```python
from build123d import *

# Parameters (mm, degrees)
F0_R      = 14
F1_DEPTH  = 15
F2_R      = 3
F3_DEPTH  = 50
F6_DEPTH  = 19.3
F7_DEPTH  = 19.3
F9_DEPTH  = 25
F10_DEPTH = 25


with BuildPart() as f1:
    # F0 (on Front) → F1 (new body)
    with BuildSketch(Plane.XZ):
        with BuildLine():
            Line((0, 44), (-94, 44))
            ThreePointArc((-94, 44), (-116, 22), (-94, 0))
            Line((-94, 0), (0, 0))
            ThreePointArc((0, 0), (22, 22), (0, 44))
        make_face()
        with BuildLine():
            Line((-105.5, 13), (-103.5, 13))
            ThreePointArc((-103.5, 13), (-101, 10.5), (-103.5, 8))
            Line((-103.5, 8), (-105.5, 8))
            ThreePointArc((-105.5, 8), (-108, 10.5), (-105.5, 13))
        make_face(mode=Mode.SUBTRACT)
        with BuildLine():
            Line((-84.5, 14), (-82.5, 14))
            ThreePointArc((-82.5, 14), (-80, 11.5), (-82.5, 9))
            Line((-82.5, 9), (-84.5, 9))
            ThreePointArc((-84.5, 9), (-87, 11.5), (-84.5, 14))
        make_face(mode=Mode.SUBTRACT)
        with BuildLine():
            Line((-96, 27), (-92, 27))
            ThreePointArc((-92, 27), (-87, 22), (-92, 17))
            Line((-92, 17), (-96, 17))
            ThreePointArc((-96, 17), (-100.999999, 22), (-96, 27))
        make_face(mode=Mode.SUBTRACT)
        with BuildLine():
            Line((-105.5, 35), (-103.5, 35))
            ThreePointArc((-103.5, 35), (-101, 32.5), (-103.5, 30))
            Line((-103.5, 30), (-105.5, 30))
            ThreePointArc((-105.5, 30), (-108, 32.5), (-105.5, 35))
        make_face(mode=Mode.SUBTRACT)
        with BuildLine():
            Line((-84.5, 35), (-82.5, 35))
            ThreePointArc((-82.5, 35), (-80, 32.5), (-82.5, 30))
            Line((-82.5, 30), (-84.5, 30))
            ThreePointArc((-84.5, 30), (-87, 32.5), (-84.5, 35))
        make_face(mode=Mode.SUBTRACT)
        with Locations((0, 22)):
            Circle(F0_R, mode=Mode.SUBTRACT)
    extrude(amount=-F1_DEPTH)

    # F2 (on Top) → F3 (cut)
    with BuildSketch(Plane.XY):
        with Locations((0, 7.5)):
            Circle(F2_R)
    extrude(amount=F3_DEPTH, mode=Mode.SUBTRACT)

    # F5 (on offset) → F6 (cut)
    with BuildSketch(Plane.XY.offset(22)):
        Polygon((4.767146, 4.243061), (5.204165, 10), (0.437019, 13.256939), (-4.767146, 10.756939), (-5.204165, 5), (-0.437019, 1.743061), align=None)
    extrude(amount=F6_DEPTH, mode=Mode.SUBTRACT)

    # F5 (on offset) → F7 (cut)
    with BuildSketch(Plane.XY.offset(22)):
        Polygon((4.767146, 4.243061), (5.204165, 10), (0.437019, 13.256939), (-4.767146, 10.756939), (-5.204165, 5), (-0.437019, 1.743061), align=None)
    extrude(amount=-F7_DEPTH, mode=Mode.SUBTRACT)

    # F8 (on offset) → F9 (cut)
    with BuildSketch(Plane.XY.offset(22)):
        Polygon((-116, 15), (-116, 7.5), (-66, 7.5), (-31, 15), align=None)
    extrude(amount=-F9_DEPTH, mode=Mode.SUBTRACT)

    # F8 (on offset) → F10 (cut)
    with BuildSketch(Plane.XY.offset(22)):
        Polygon((-116, 15), (-116, 7.5), (-66, 7.5), (-31, 15), align=None)
    extrude(amount=F10_DEPTH, mode=Mode.SUBTRACT)


solid = f1.part
```
For this review, take the finished solid that the model builds, in its own axes (mm). A direction names the side the tool comes from. Coordinates: 2 decimals unless noted, no trailing zeros. Loops run counter-clockwise (first coordinate to the right, second up) from the corner with the lowest first, then second, coordinate; pieces in that order, holes last.
1. Insertion check: P1, Ø2, axis at x = -99.5, z = 23, coming from the -Y side; P2, Ø5, axis at y = 2, z = 29, coming from the -X side; P3, Ø0.6, axis at x = -105, y = 2.5, coming from the -Z side; P4, Ø5, axis at x = -101, z = 23.5, coming from the +Y side. Each pin has a flat end and moves straight along its axis. Give the tip position at first contact, or say it passes through.
2. Add section D-D, the plane z = 39. Give the boundary of the cut face in (x, y), then the cut area to 3 significant figures.
3. Add section A-A, the plane z = 22. Give the boundary of the cut face in (x, y), then the cut area to 3 significant figures.
4. For line 1 (Y direction, x = 0, z = 1); line 2 (X direction, y = 5.5, z = 26); line 3 (Y direction, x = -4.5, z = 38), list the stretches that pass through material, from the lowest coordinate up.
5. Mouldability with a two-part tool opening along Y and no side actions: class faces 1 (the flat face through (4.983, 7.081, 38.104)), 2 (the flat face through (-37, 6, 0)), 3 (the flat face through (-48, 0, 22)) as +Y half, -Y half, draft (parallel to the pull), parting line (faces both ways), or undercut.
6. For faces 4 (the flat face through (2, 5, 41.3)), 5 (the cylindrical face through (-101, 4, 22)), 6 (the cylindrical face through (-3, 7.6, 42.6)), list the 3-axis set-ups (+Z, -Z, +X, -X, +Y, -Y) from which the entire face can be reached by the end or side of a thin tool; tool diameter is ignored.
7. Add section B-B, the plane z = 11.5. Give the boundary of the cut face in (x, y), then the cut area to 3 significant figures.
8. Add section C-C, the plane x = -59. Give the boundary of the cut face in (y, z), then the cut area to 3 significant figures.
Result:
1. P1: passes through
1. P2: stops at x = -115.53
1. P3: stops at z = 2.78
1. P4: stops at y = 7.5
2. outline: (-107.96, 0) - (13.96, 0) - (13.96, 15) - (-31, 15) - (-66, 7.5) - (-107.96, 7.5) - close; hole (-5.2, 5) - (-0.44, 1.74) - (4.77, 4.24) - (5.2, 10) - (0.44, 13.26) - (-4.77, 10.76) - close
2. area: 1,300 mm2
3. outline: (-116, 0) - (-101, 0) - (-101, 7.5) - (-116, 7.5) - close; (-87, 0) - (-14, 0) - (-14, 15) - (-31, 15) - (-66, 7.5) - (-87, 7.5) - close; (14, 0) - (22, 0) - (22, 15) - (14, 15) - close
3. area: 1,040 mm2
4. line 1: y = 0 to 4.5, 10.5 to 15
4. line 2: x = -115.63 to -99, -89 to -13.42, 13.42 to 21.63
4. line 3: y = 0 to 4.52, 10.89 to 15
5. face 1: undercut
5. face 2: draft
5. face 3: -Y half
6. face 4: none
6. face 5: +Y, -Y
6. face 6: +Z, -Z
7. outline: (-113.33, 0) - (-107.79, 0) - (-107.79, 7.5) - (-113.33, 7.5) - close; (-101.21, 0) - (-87, 0) - (-87, 7.5) - (-101.21, 7.5) - close; (-80, 0) - (-9.26, 0) - (-9.26, 15) - (-31, 15) - (-66, 7.5) - (-80, 7.5) - close; (9.26, 0) - (19.33, 0) - (19.33, 15) - (9.26, 15) - close
7. area: 1,120 mm2
8. outline: (0, 0) - (9, 0) - (9, 44) - (0, 44) - close
8. area: 396 mm2
